Model file for the job. Use its own axes, mm. Face numbers are marked on the shaded views. A direction names the side the tool comes from. Round coordinates to 2 decimals unless told otherwise and drop trailing zeros. Order: outer loops, then holes, each group sorted by start corner. A loop starts at its lowest first (then second) coordinate and runs counter-clockwise, first axis right, second up. Notation, with made-up numbers: (-2.75, 10) -> (30.25, 10) arc R21 cw to (30.25, 20) -> close; hole circle Ø3 at (-38, 73.25). An arc over 180 degrees is marked (long way). Answer as CSV lines item,"result".
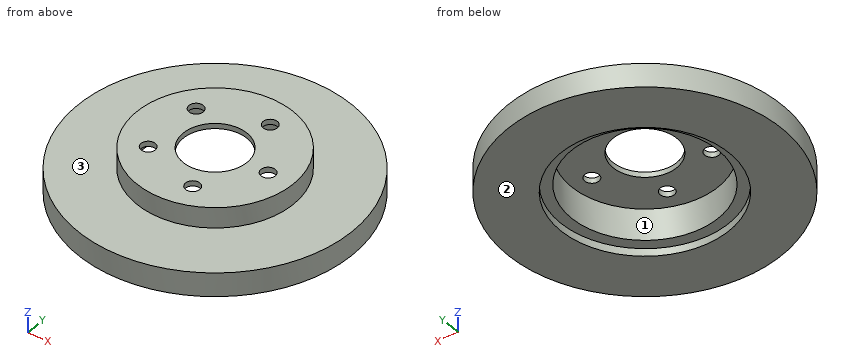
```python
from build123d import *

# Parameters (mm, degrees)
F0_R     = 144
F1_DEPTH = 25
F2_R     = 82.3
F3_DEPTH = 21.5
F4_R     = 77.15
F5_DEPTH = 41
F6_R     = 88.5
F7_DEPTH = 8
F8_R     = 33.5
F8_R_2   = 7.5
F9_DEPTH = 25


with BuildPart() as f1:
    # F0 (on Top) → F1 (new body)
    with BuildSketch(Plane.XY):
        Circle(F0_R)
    extrude(amount=F1_DEPTH)

    # F2 (on face) → F3 (join)
    with BuildSketch(Plane.XY.offset(25)):
        Circle(F2_R)
    extrude(amount=F3_DEPTH)

    # F4 (on face) → F5 (cut)
    with BuildSketch(Plane(origin=(0, 0, 0), x_dir=(1, 0, 0), z_dir=(0, 0, -1))):
        Circle(F4_R)
    extrude(amount=-F5_DEPTH, mode=Mode.SUBTRACT)

    # F6 (on face) → F7 (cut)
    with BuildSketch(Plane(origin=(0, 0, 0), x_dir=(1, 0, 0), z_dir=(0, 0, -1))):
        Circle(F6_R)
    extrude(amount=-F7_DEPTH, mode=Mode.SUBTRACT)

    # F8 (on face) → F9 (cut)
    with BuildSketch(Plane.XY.offset(46.5)):
        Circle(F8_R)
        with Locations((56, 0)):
            Circle(F8_R_2)
        with Locations((17.304952, 53.259165)):
            Circle(F8_R_2)
        with Locations((-45.304952, 32.915974)):
            Circle(F8_R_2)
        with Locations((-45.304952, -32.915974)):
            Circle(F8_R_2)
        with Locations((17.304952, -53.259165)):
            Circle(F8_R_2)
    extrude(amount=-F9_DEPTH, mode=Mode.SUBTRACT)


solid = f1.part
```
Q1. Saw through at D-D (y = -68.5). Write the cut outline in (x, z).
Checks:
outline,"(-126.66, 0) -> (-56.04, 0) -> (-56.04, 8) -> (-35.49, 8) -> (-35.49, 41) -> (35.49, 41) -> (35.49, 8) -> (56.04, 8) -> (56.04, 0) -> (126.66, 0) -> (126.66, 25) -> (45.62, 25) -> (45.62, 46.5) -> (-45.62, 46.5) -> (-45.62, 25) -> (-126.66, 25) -> close"
Q2. Wall check: L1, parallel to X at y = 1, z = 3.5; L2, parallel to Y at x = 0, z = 26; L3, parallel to Z at x = 27, y = -84.5. Give the ranges that are in metal, low to high. Write a range as [from, to].
Checks:
L1,"[-144, -88.49], [88.49, 144]"
L2,"[-82.3, -77.15], [77.15, 82.3]"
L3,"[0, 25]"
Q3. Flat gauge pins, fed straight in: pin 1 (17 mm diameter, centred on x = 17.3, y = 53.26, fed in from -Z); pin 2 (12 mm diameter, centred on y = 25, z = 32, fed in from -X); pin 3 (5 mm diameter, centred on x = 37.5, y = 107, fed in from +Z); pin 4 (12 mm diameter, centred on x = -45.3, y = -32.92, fed in from -Z). Where does each tip first touch, or does it go through?
Checks:
pin 1,"z = 41"
pin 2,"x = -80.08"
pin 3,"z = 25"
pin 4,"through"
Q4. Saw through at B-B (y = 0). Write the cut outline in (x, z), plus the area to 3 significant figures.
Checks:
outline,"(-144, 0) -> (-88.5, 0) -> (-88.5, 8) -> (-77.15, 8) -> (-77.15, 41) -> (-33.5, 41) -> (-33.5, 46.5) -> (-82.3, 46.5) -> (-82.3, 25) -> (-144, 25) -> close; (33.5, 41) -> (48.5, 41) -> (48.5, 46.5) -> (33.5, 46.5) -> close; (63.5, 41) -> (77.15, 41) -> (77.15, 8) -> (88.5, 8) -> (88.5, 0) -> (144, 0) -> (144, 25) -> (82.3, 25) -> (82.3, 46.5) -> (63.5, 46.5) -> close"
area,"3,780 mm²"
Q5. Saw through at C-C (z = 31.5). Write the cut outline in (x, y), plus the area to 3 significant figures.
Checks:
outline,"circle Ø164.6 at (0, 0); hole circle Ø154.3 at (0, 0)"
area,"2,580 mm²"
Q6. Tool access for the marked faces 1, 2 and 3: list every direction of +Z, -Z, +X, -X, +Y, -Y with a clear straight run to the whole face (end or side of a thin tool).
Checks:
face 1,"-Z"
face 2,"-Z, +X, -X, +Y, -Y"
face 3,"+Z"
Q7. Saw through at A-A (x = 0). Write the cut outline in (y, z).
Checks:
outline,"(-144, 0) -> (-88.5, 0) -> (-88.5, 8) -> (-77.15, 8) -> (-77.15, 41) -> (-33.5, 41) -> (-33.5, 46.5) -> (-82.3, 46.5) -> (-82.3, 25) -> (-144, 25) -> close; (33.5, 41) -> (77.15, 41) -> (77.15, 8) -> (88.5, 8) -> (88.5, 0) -> (144, 0) -> (144, 25) -> (82.3, 25) -> (82.3, 46.5) -> (33.5, 46.5) -> close"
